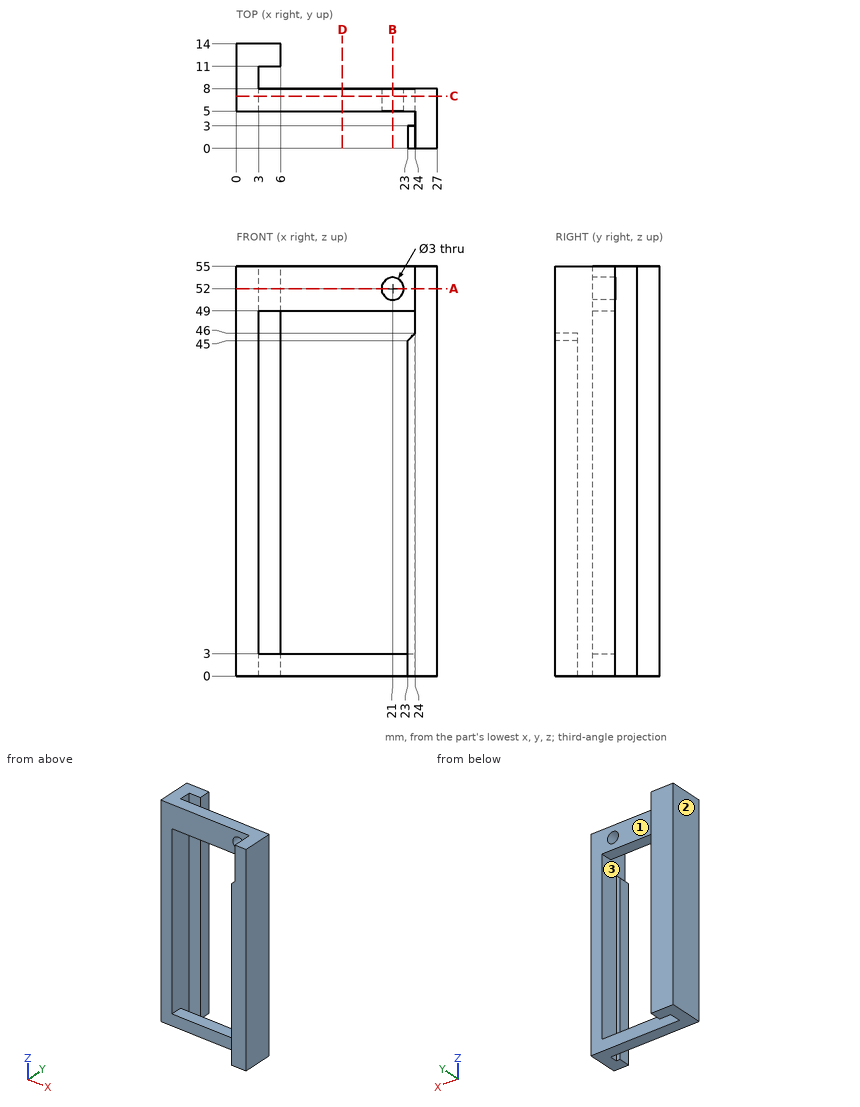
Input: dimensioned drawing with shaded views. Units: mm. Origin: part minimum x, y, z. Give positions to 0.01 mm unless a question says otherwise; leave off trailing zeros. Write each loop counter-clockwise with the first axis right and the second up, starting at its lowest first coordinate (ties: lowest second). Pieces come first, ordered by that corner, then holes.
Q1. Section B-B, the plane x = 21. Output: boundary loops of the cut face in (y, z), plus the area to 3 significant figures.
Q2. Section C-C, the plane y = 7. Output: boundary loops of the cut face in (x, z), plus the area to 3 significant figures.
Q3. Material intervals for probe 1 along Z at (x, y) = (21, 6.95); probe 2 along X at (y, z) = (5.75, 19); probe 3 along Z at (x, y) = (16.5, 7.5), sorted ascending.
Q4. Section A-A, the plane z = 52. Output: boundary loops of the cut face in (x, y).
Q5. Section D-D, the plane x = 14.25. Output: boundary loops of the cut face in (y, z).
Q6. First-contact query: P1, Ø8, axis at x = 13.5, z = 47.5, coming from the +Y side; P2, Ø4, axis at x = 6, z = 38.5, coming from the -Y side; P3, Ø3.5, axis at x = 4, z = 24.5, coming from the -Y side; P4, Ø12, axis at x = 15.5, z = 31, coming from the +Y side. Flat tips, straight axial feed; report the tip coordinate or a pass-through.
Q7. Pull-direction query (X, two-part tool) for the marked faces 1, 2 and 3; classes: pulls with the +X half, pulls with the -X half, needs draft (parallel to the pull), parting line crosses it, or undercut.
Filled in:
1. outline: (5, 0) - (8, 0) - (8, 3) - (5, 3) - close; (5, 49) - (8, 49) - (8, 50.5) - (5, 50.5) - close; (5, 53.5) - (8, 53.5) - (8, 55) - (5, 55) - close
1. area: 18.0 mm2
2. outline: (0, 0) - (27, 0) - (27, 55) - (0, 55) - close; hole (3, 3) - (24, 3) - (24, 49) - (3, 49) - close; hole circle Ø3 at (21, 52)
2. area: 512 mm2
3. probe 1: z = 0 to 3, 49 to 50.5, 53.5 to 55
3. probe 2: x = 0 to 3, 24 to 27
3. probe 3: z = 0 to 3, 49 to 55
4. outline: (0, 5) - (19.5, 5) - (19.5, 8) - (3, 8) - (3, 11) - (6, 11) - (6, 14) - (0, 14) - close; (22.5, 5) - (24, 5) - (24, 0) - (27, 0) - (27, 8) - (22.5, 8) - close
5. outline: (5, 0) - (8, 0) - (8, 3) - (5, 3) - close; (5, 49) - (8, 49) - (8, 55) - (5, 55) - close
6. P1: stops at y = 8
6. P2: stops at y = 11
6. P3: stops at y = 5
6. P4: passes through
7. face 1: needs draft
7. face 2: pulls with the -X half
7. face 3: undercut
